```python
from build123d import *

# Parameters (mm, degrees)
SKETCH1_W           = 35.56
SKETCH1_H           = 5.08
BOSS_EXTRUDE1_DEPTH = 92.202
SKETCH4_W           = 10.16
SKETCH4_H           = 2.54
BOSS_EXTRUDE4_DEPTH = 5.08
CUT_EXTRUDE1_DEPTH  = 2.54
CUT_EXTRUDE3_DEPTH  = 95.037990217
SKETCH13_R          = 1.5875
CUT_EXTRUDE4_DEPTH  = 95.037990217


with BuildPart() as part:
    # Sketch1 → Boss-Extrude1 (new body)
    with BuildSketch(Plane(origin=(0, 0, 0), x_dir=(1, 0, 0), z_dir=(0, 1, 0))):
        Rectangle(SKETCH1_W, SKETCH1_H)
    extrude(amount=BOSS_EXTRUDE1_DEPTH)

    # Sketch4 → Boss-Extrude4 (add)
    with BuildSketch(Plane.XY.offset(2.54)):
        with Locations((-12.7, 90.932)):
            Rectangle(SKETCH4_W, SKETCH4_H)
    extrude(amount=BOSS_EXTRUDE4_DEPTH)

    # Sketch5 → Cut-Extrude1 (cut)
    with BuildSketch(Plane(origin=(0, 92.202, 0), x_dir=(1, 0, 0), z_dir=(0, 1, 0))):
        with BuildLine():
            ThreePointArc((-12.7, -7.62), (-16.292102448, -6.132102448), (-17.78, -2.54))
            Line((-17.78, -2.54), (-17.78, -7.62))
            Line((-17.78, -7.62), (-12.7, -7.62))
        make_face()
        with BuildLine():
            Line((-7.62, -7.62), (-7.62, -2.54))
            ThreePointArc((-7.62, -2.54), (-9.107897552, -6.132102448), (-12.7, -7.62))
            Line((-12.7, -7.62), (-7.62, -7.62))
        make_face()
    extrude(amount=-CUT_EXTRUDE1_DEPTH, mode=Mode.SUBTRACT)

    # Sketch7 → Cut-Extrude3 (cut, through all)
    with BuildSketch(Plane.XY.offset(2.54)):
        with BuildLine():
            ThreePointArc((-12.7, 0), (-3.575035086, 44.457914169), (-7.62, 89.662))
            Line((-7.62, 89.662), (-17.78, 89.662))
            Line((-17.78, 89.662), (-17.78, 0))
            Line((-17.78, 0), (-12.7, 0))
        make_face()
        with BuildLine():
            ThreePointArc((17.78, 88.831864431), (9.052257411, 42.18144567), (-12.7, 0))
            Line((-12.7, 0), (17.78, 0))
            Line((17.78, 0), (17.78, 88.831864431))
        make_face()
    extrude(amount=-CUT_EXTRUDE3_DEPTH, mode=Mode.SUBTRACT)

    # Sketch13 → Cut-Extrude4 (cut, through all)
    with BuildSketch(Plane.XY.offset(2.54)):
        with Locations((3.446895522, 39.620022835)):
            Circle(SKETCH13_R)
    extrude(amount=-CUT_EXTRUDE4_DEPTH, mode=Mode.SUBTRACT)


solid = part.part
```
Geometry: final body of the model. Coordinates: model frame, mm. A direction names the side the tool comes from. Coordinates: 2 decimals unless noted, no trailing zeros. Write each loop counter-clockwise with the first axis right and the second up, starting at its lowest first coordinate (ties: lowest second). Pieces come first, ordered by that corner, then holes. Notation, with made-up numbers: M -4.5,73.25 L 11.5,73.25 A27 cw 11.5,111.25 Z; hole C 74,-32 d6. An arc over 180 degrees is marked long. Use CSV: the item, a comma, the result in double quotes. Start each with the question number.
1. Cut plane D-D on y = 72. Return the cut outline in (x, z).
2. Reachability of faces 1 (the face through (-13, 89.662, 3)), 2 (the face through (17.78, 90, 0)) from +Z, -Z, +X, -X, +Y, -Y: full face, straight path, thin tool, end or side. Return the list, or none.
3. Cut plane A-A on x = -11.5. Return the cut outline in (y, z), plus the area to 3 significant figures.
4. Ray query, probe 1 along Y at (x, z) = (-14, 6); probe 2 along Z at (x, y) = (2.5, 87); probe 3 along Y at (x, z) = (4, -2). Return the intervals inside material, ascending.
5. First-contact query: P1, Ø3, axis at y = 65, z = 0.5, coming from the -X side; P2, Ø10, axis at x = -3, y = 32.5, coming from the +Z side; P3, Ø5, axis at y = 82.5, z = -1.5, coming from the +X side. Flat tips, straight axial feed; report the tip coordinate or a pass-through.
6. Cut plane C-C on x = -6. Return the cut outline in (y, z).
7. Cut plane B-B on z = 0.5. Return the cut outline in (x, y) (1 decimal).
8. Mould query, pull axis Y, two halves, no side actions, for faces 3 (the face through (4, 56, -2.54)), 4 (the face through (-3.612, 43.821, 0.036)), 5 (the face through (3.1, 38.07, 0.04)), 6 (the face through (-4, 92.202, 1)). Classes: pulls with the +Y half, pulls with the -Y half, needs draft (parallel to the pull), parting line crosses it, or undercut.
Entries:
1,outline,"M -4.45,-2.54 L 16.24,-2.54 L 16.24,2.54 L -4.45,2.54 Z"
2,face 1,"+Z, -Z, -X"
2,face 2,"+Z, -Z, +X, +Y, -Y"
3,outline,"M 1.7,-2.54 L 3.43,-2.54 L 3.43,2.54 L 1.7,2.54 Z; M 89.66,-2.54 L 92.2,-2.54 L 92.2,7.48 L 89.66,7.48 Z"
3,area,"34.2 mm²"
4,probe 1,"89.66 to 92.2"
4,probe 2,"-2.54 to 2.54"
4,probe 3,"29.27 to 38.13, 41.11 to 92.2"
5,P1,"x = -3.88"
5,P2,"z = 2.54"
5,P3,"x = 17.58"
6,outline,"M 10.12,-2.54 L 24.51,-2.54 L 24.51,2.54 L 10.12,2.54 Z; M 82.07,-2.54 L 92.2,-2.54 L 92.2,2.54 L 82.07,2.54 Z"
7,outline,"M -17.8,89.7 L -7.6,89.7 A156.1 cw -12.7,0 A163.6 ccw 17.8,88.8 L 17.8,92.2 L -17.8,92.2 Z; hole C 3.4,39.6 d3.2"
8,face 3,"needs draft"
8,face 4,"undercut"
8,face 5,"undercut"
8,face 6,"pulls with the +Y half"
